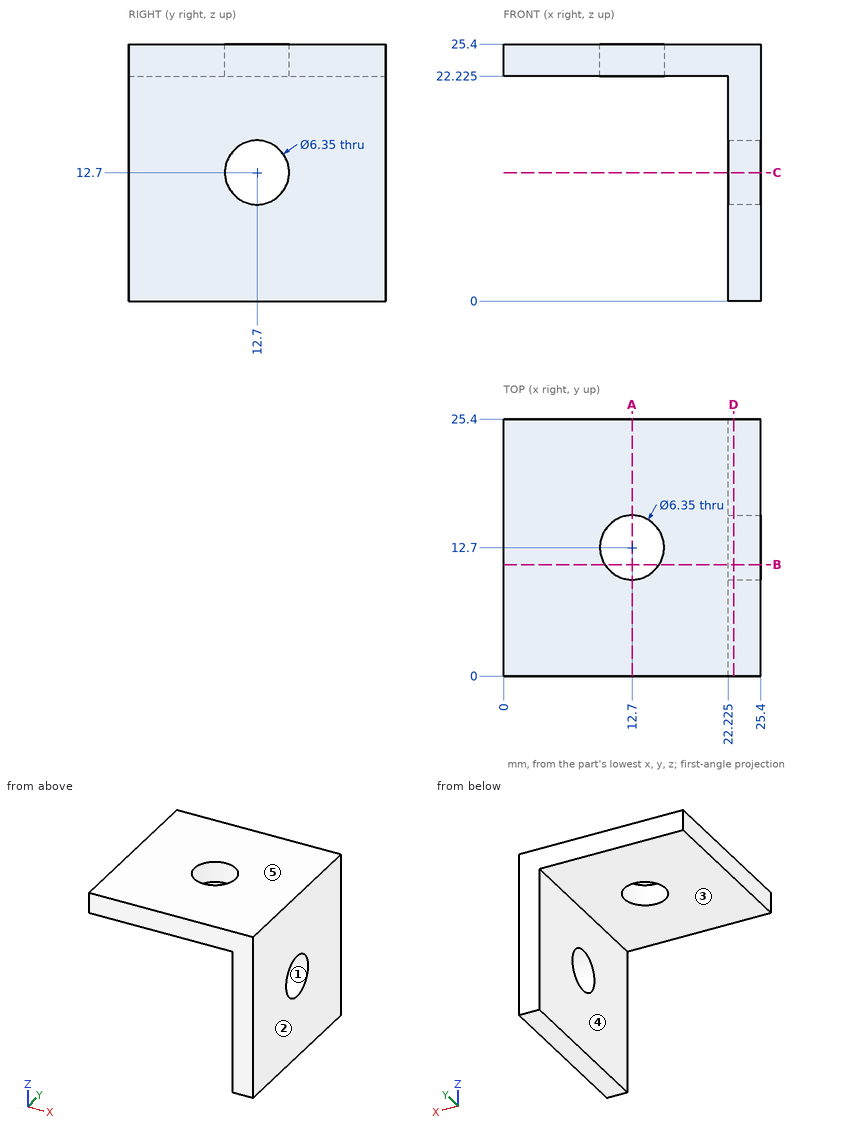
The figure shows three views and two pictorial views of one solid part (mm, origin at its lowest corner). Answer the questions. A direction names the side the tool comes from. Give positions to 0.01 mm unless a question says otherwise; leave off trailing zeros. Write each loop counter-clockwise with the first axis right and the second up, starting at its lowest first coordinate (ties: lowest second). Pieces come first, ordered by that corner, then holes.
Q1. For a pull along Z with two mould halves and no side action, classify the marked faces 1, 2 and 3 as released by +Z, released by -Z, zero draft, split by the parting line, or undercut.
Answer:
face 1: undercut
face 2: zero draft
face 3: released by -Z
Q2. A tool of negligible diameter and unlimited length cuts with its end or side. For the marked faces 4 and 5, from which of +Z, -Z, +X, -X, +Y, -Y can it reach the whole face along a straight path? Write none if from no direction.
Answer:
face 4: -Z, -X, +Y, -Y
face 5: +Z, +X, -X, +Y, -Y
Q3. The part is cut by section B-B on y = 11. Give the vertices of the cut face in (x, z) (3 decimals), and give its area (3 significant figures).
Answer:
outline: (0, 22.225) - (10.018, 22.225) - (10.018, 25.4) - (0, 25.4) - close; (15.382, 22.225) - (22.225, 22.225) - (22.225, 15.382) - (25.4, 15.382) - (25.4, 25.4) - (15.382, 25.4) - close; (22.225, 0) - (25.4, 0) - (25.4, 10.018) - (22.225, 10.018) - close
area: 117 mm2
Q4. The part is cut by section C-C on z = 12.7. Give the vertices of the cut face in (x, y) (3 decimals), and give its area (3 significant figures).
Answer:
outline: (22.225, 0) - (25.4, 0) - (25.4, 9.525) - (22.225, 9.525) - close; (22.225, 15.875) - (25.4, 15.875) - (25.4, 25.4) - (22.225, 25.4) - close
area: 60.5 mm2
Q5. Straight lines are drawn through the part: L1, parallel to Y at x = 24.3, z = 12.7 (3 decimals); L2, parallel to Z at x = 2.5, y = 8.25 (3 decimals). For each, find the intervals that lie inside material, in ascending order.
Answer:
L1: y = 0 to 9.525, 15.875 to 25.4
L2: z = 22.225 to 25.4
Q6. Given pin 1 (6.5 mm diameter, centred on x = 9.5, y = 7.5, fed in from -Z) (3 decimals); pin 2 (10 mm diameter, centred on y = 12.7, z = 12.7, fed in from -X) (3 decimals), each flat-ended and moving along its own axis, determine where each tip first touches the part or whether it passes through.
Answer:
pin 1: stops at z = 22.225
pin 2: stops at x = 22.225
Q7. The part is cut by section D-D on x = 22.75. Give the vertices of the cut face in (y, z) (3 decimals).
Answer:
outline: (0, 0) - (25.4, 0) - (25.4, 25.4) - (0, 25.4) - close; hole circle Ø6.35 at (12.7, 12.7)
Q8. The part is cut by section A-A on x = 12.7. Give the vertices of the cut face in (y, z) (3 decimals).
Answer:
outline: (0, 22.225) - (9.525, 22.225) - (9.525, 25.4) - (0, 25.4) - close; (15.875, 22.225) - (25.4, 22.225) - (25.4, 25.4) - (15.875, 25.4) - close
